For this review, take the finished solid that the model builds, in its own axes (mm). Face numbers are marked on the shaded views. A direction names the side the tool comes from. Give positions to 0.01 mm unless a question says otherwise; leave off trailing zeros. Order: outer loops, then holes, each group sorted by start corner. A loop starts at its lowest first (then second) coordinate and runs counter-clockwise, first axis right, second up. Notation, with made-up numbers: (-12, 78.5) - (7, 78.5) arc R22 ccw to (7, 115.5) - close; hole circle Ø9 at (72, -7). An arc over 180 degrees is marked (long way). Use a Markdown table: item, result. Add a question column.
1) We need section A-A on y = -2. Write out the cut boundary in (x, z).
2) Clearance check with flat-ended pins moving along their axes: P1, Ø22.5, axis at y = 7, z = -20, coming from the +X side; P2, Ø12, axis at x = -6, y = -48, coming from the -Z side; P3, Ø5, axis at y = 46.5, z = -67.5, coming from the +X side; P4, Ø12, axis at x = 103, y = 8, coming from the -Z side. State where each tip first meets the part, or that it passes through.
3) Machinability: for the marked faces 1, 2 and 3, which of the approach directions +Z, -Z, +X, -X, +Y, -Y give a long, thin tool a straight path to every point of the face, cutting with its end or side? Answer none if there is none.
4) We need section D-D on x = 86.5. Write out the cut boundary in (y, z), then the cut area to 3 significant figures.
5) Mouldability with a two-part tool opening along Y and no side actions: class the marked faces 4, 5 and 6 as released by +Y, released by -Y, zero draft, split by the parting line, or undercut.
6) We need section C-C on x = 18.5. Write out the cut boundary in (y, z), then the cut area to 3 significant figures.
7) Wall thickness on L1, parallel to Z at x = 28, y = -16; L2, parallel to Z at x = -27, y = 43; L3, parallel to Z at x = 41, y = -48: over which ranges is each line inside the solid? List them lowest first.
8) We need section B-B on z = -12. Write out the cut boundary in (x, y).
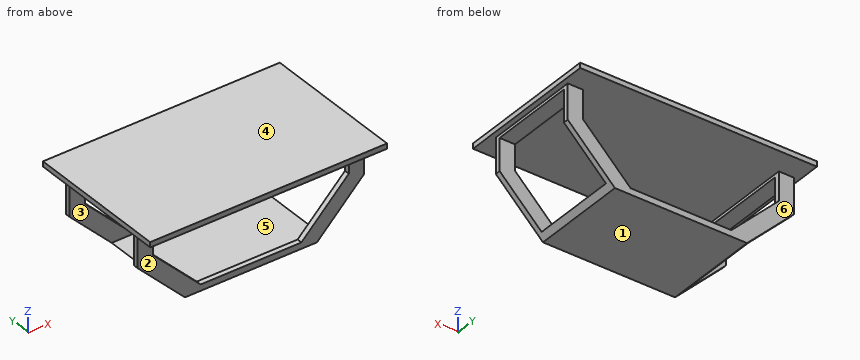
```python
from build123d import *

# Parameters (mm, degrees)
SKETCH1_W           = 230
SKETCH1_H           = 140
BOSS_EXTRUDE1_DEPTH = 5
SKETCH4_W           = 15
SKETCH4_H           = 94
CUT_EXTRUDE1_DEPTH  = 118
SKETCH7_W           = 72
SKETCH7_H           = 84
CUT_EXTRUDE2_DEPTH  = 226


with BuildPart() as part:
    # Sketch1 → Boss-Extrude1 (new body)
    with BuildSketch(Plane.XY):
        Rectangle(SKETCH1_W, SKETCH1_H)
    extrude(amount=BOSS_EXTRUDE1_DEPTH)

    # Sweep3: sweep along a path in Sketch5
    with BuildLine(Plane(origin=(0, 0, 0), x_dir=(1, 0, 0), z_dir=(0, 1, 0))) as sweep3_path:
        Line((-100, 0), (-100, 30))
        Line((-100, 30), (-60, 70))
        Line((-60, 70), (60, 70))
        Line((60, 70), (100, 30))
        Line((100, 30), (100, 0))
    # Sketch4 → Sweep3 (sweep)
    with BuildSketch(Plane.XY):
        with Locations((-102.5, 0)):
            Rectangle(SKETCH4_W, SKETCH4_H)
    sweep(path=sweep3_path.line, transition=Transition.RIGHT)

    # Sketch6 → Cut-Extrude1 (cut, through all)
    with BuildSketch(Plane(origin=(0, 47, 0), x_dir=(1, 0, 0), z_dir=(0, 1, 0))):
        Polygon((-48.928932188, 74), (48.928932188, 74), (76.464466094, 46.464466094), (-76.464466094, 46.464466094), align=None)
    extrude(amount=-CUT_EXTRUDE1_DEPTH, mode=Mode.SUBTRACT)

    # Sketch7 → Cut-Extrude2 (cut, through all)
    with BuildSketch(Plane.ZY.offset(110)):
        with Locations((-39, 0)):
            Rectangle(SKETCH7_W, SKETCH7_H)
    extrude(amount=-CUT_EXTRUDE2_DEPTH, mode=Mode.SUBTRACT)


solid = part.part
```
Checked values:
| question | item | result |
|---|---|---|
| 1 | outline | (-115, 0) - (-110, 0) - (-110, -3) - (-95, -3) - (-95, 0) - (95, 0) - (95, -3) - (110, -3) - (110, 0) - (115, 0) - (115, 5) - (-115, 5) - close; (-69.14, -75) - (-64.14, -80) - (64.14, -80) - (69.14, -75) - close |
| 2 | P1 | through |
| 2 | P2 | z = -80 |
| 2 | P3 | x = 79.14 |
| 2 | P4 | z = -3 |
| 3 | face 1 | -Z, +X, -X, +Y, -Y |
| 3 | face 2 | -Z, +X, -X, -Y |
| 3 | face 3 | +X, -X |
| 4 | outline | (-70, 0) - (70, 0) - (70, 5) - (-70, 5) - close; (-47, -57.64) - (-42, -57.64) - (-42, -36.43) - (-47, -36.43) - close; (42, -57.64) - (47, -57.64) - (47, -36.43) - (42, -36.43) - close |
| 4 | area | 912 mm² |
| 5 | face 4 | zero draft |
| 5 | face 5 | undercut |
| 5 | face 6 | released by +Y |
| 6 | outline | (-70, 0) - (70, 0) - (70, 5) - (-70, 5) - close; (-47, -80) - (47, -80) - (47, -74) - (42, -74) - (42, -75) - (-42, -75) - (-42, -74) - (-47, -74) - close |
| 6 | area | 1,180 mm² |
| 7 | L1 | -80 to -75, 0 to 5 |
| 7 | L2 | -80 to -74, 0 to 5 |
| 7 | L3 | 0 to 5 |
| 8 | outline | (-110, -47) - (-95, -47) - (-95, -42) - (-110, -42) - close; (-110, 42) - (-95, 42) - (-95, 47) - (-110, 47) - close; (95, -47) - (110, -47) - (110, -42) - (95, -42) - close; (95, 42) - (110, 42) - (110, 47) - (95, 47) - close |
